from build123d import *

# Parameters (mm, degrees)
BOX001_W      = 10
BOX001_H      = 10
BOX001_DEPTH  = 8
EXTRUDE_DEPTH = 10
BOX_W         = 16
BOX_H         = 16
BOX_DEPTH     = 10


with BuildPart() as cube001:
    # Box001 → Box001 (new body)
    with BuildSketch(Plane(origin=(-5, -5, 0), x_dir=(1, 0, 0), z_dir=(0, 0, 1))):
        with Locations((5, 5)):
            Rectangle(BOX001_W, BOX001_H)
    extrude(amount=BOX001_DEPTH)


with BuildPart() as extrude_body:
    # Sketch → Extrude (new body)
    with BuildSketch(Plane.XY):
        with BuildLine():
            Line((1.12075, 2.839983), (-4.120749, 1.699111))
            Line((-4.371559, -0.236927), (-4.120749, 1.699111))
            Line((-4.371559, -0.236927), (-3.566567, -0.41805))
            ThreePointArc((-0.915655, 0.079537), (-2.453717, 0.963407), (-3.566567, -0.41805))
            Line((-0.411383, -1.079694), (-0.915655, 0.079537))
            ThreePointArc((-0.411383, -1.079694), (1.076577, -1.73701), (2.017311, -0.409942))
            Line((0.800522, 0.990688), (2.017311, -0.409942))
            Line((2.605595, 1.358264), (0.800522, 0.990688))
            Line((1.12075, 2.839983), (2.605595, 1.358264))
        make_face()
    extrude(amount=EXTRUDE_DEPTH)


with BuildPart() as extrude_body_1:
    # Extrude placement: moved
    add(extrude_body.part.moved(Location((1, -0.5, 10))))


with BuildPart() as cut:
    # Box → Box (new body)
    with BuildSketch(Plane(origin=(-8, -8, 0), x_dir=(1, 0, 0), z_dir=(0, 0, 1))):
        with Locations((8, 8)):
            Rectangle(BOX_W, BOX_H)
    extrude(amount=BOX_DEPTH)

    # Fusion: union Extrude body
    add(extrude_body_1.part)

    # Cut: cut Cube001
    add(cube001.part, mode=Mode.SUBTRACT)


solid = cut.part
Work out the finished part from the listing and answer in its coordinate system (mm). A direction names the side the tool comes from. Give positions to 0.01 mm unless a question says otherwise; leave off trailing zeros. Order: outer loops, then holes, each group sorted by start corner. A loop starts at its lowest first (then second) coordinate and runs counter-clockwise, first axis right, second up. Notation, with made-up numbers: (57, -26.5) -> (67, -26.5) arc R9 ccw to (67, -19.5) -> close; hole circle Ø1 at (83.5, 60.5). An arc over 180 degrees is marked (long way). One line per item, written item: value.
Item 1: Flat-ended cylindrical pins translate along their axes: P1, Ø2, axis at x = 2.5, z = 16.5, coming from the +Y side; P2, Ø1, axis at x = 0, z = 17.5, coming from the -Y side; P3, Ø6, axis at y = 1.5, z = 14, coming from the -X side. Find the tip coordinate at first contact, or state that the pin passes through.
Answer sheet:
P1: y = 2.34
P2: y = -1.38
P3: x = -3.37
Item 2: Determine the mould class of faces 1 (the cylindrical face through (2.053, -2.243, 14.93)), 2 (the flat face through (0, 8, 5)), 3 (the flat face through (5, 0, 4)) for opening direction X: released by +X, released by -X, zero draft, split by the parting line, or undercut.
Answer sheet:
face 1: split by the parting line
face 2: zero draft
face 3: undercut
Item 3: Find section B-B, the plane x = 4.25. Give the vertices of the cut face in (y, z).
Answer sheet:
outline: (-8, 0) -> (-5, 0) -> (-5, 8) -> (5, 8) -> (5, 0) -> (8, 0) -> (8, 10) -> (-8, 10) -> close
Item 4: A tool of negligible diameter and unlimited length cuts with its end or side. For faces 4 (the flat face through (2.716, 0.677, 14.93)), 5 (the flat face through (2.85, 1.61, 14.93)), 6 (the flat face through (0.34, -1.01, 14.93)), 7 (the flat face through (0, 0, 8)), 8 (the flat face through (-2.975, -0.826, 14.93)), from which of +Z, -Z, +X, -X, +Y, -Y can it reach the whole face along a straight path? Write none if from no direction.
Answer sheet:
face 4: +Z, +X
face 5: +Z, +X, +Y
face 6: +Z, -Y
face 7: -Z
face 8: +Z, -X, -Y
Item 5: Find section D-D, the plane z = 16. Give the vertices of the cut face in (x, y).
Answer sheet:
outline: (-3.37, -0.74) -> (-2.57, -0.92) arc R1.37 cw to (0.08, -0.42) -> (0.59, -1.58) arc R1.29 ccw to (3.02, -0.91) -> (1.8, 0.49) -> (3.61, 0.86) -> (2.12, 2.34) -> (-3.12, 1.2) -> close
Item 6: Find section A-A, the plane z = 4.5. Give the vertices of the cut face in (x, y).
Answer sheet:
outline: (-8, -8) -> (8, -8) -> (8, 8) -> (-8, 8) -> close; hole (-5, -5) -> (5, -5) -> (5, 5) -> (-5, 5) -> close
Item 7: Straight lines are drawn through the part: probe 1 along X at (y, z) = (2.25, 4); probe 2 along Z at (x, y) = (-1, -0.25). For each, find the intervals that lie inside material, in ascending order.
Answer sheet:
probe 1: -8 to -5, 5 to 8
probe 2: 8 to 10
